from build123d import *

# Parameters (mm, degrees)
SKETCH1_W           = 38.1
SKETCH1_H           = 38.1
BOSS_EXTRUDE1_DEPTH = 61.087
SKETCH2_R           = 45.085
BOSS_EXTRUDE2_DEPTH = 3.175


with BuildPart() as part:
    # Sketch1 → Boss-Extrude1 (new body)
    with BuildSketch(Plane(origin=(0, 0, 0), x_dir=(1, 0, 0), z_dir=(0, 1, 0))):
        Rectangle(SKETCH1_W, SKETCH1_H)
    extrude(amount=BOSS_EXTRUDE1_DEPTH)

    # Sketch2 → Boss-Extrude2 (add)
    with BuildSketch(Plane.XZ):
        Circle(SKETCH2_R)
    extrude(amount=BOSS_EXTRUDE2_DEPTH)


solid = part.part
Here's how the part is built. I have some questions about the finished solid (model axes, mm). A direction names the side the tool comes from. Give positions to 0.01 mm unless a question says otherwise; leave off trailing zeros. Order: outer loops, then holes, each group sorted by start corner. A loop starts at its lowest first (then second) coordinate and runs counter-clockwise, first axis right, second up. Notation, with made-up numbers: M 69.25,4.25 L 75.25,4.25 A24 ccw 75.25,40.25 Z; hole C 66,29.25 d4. An arc over 180 degrees is marked long. Answer as a JSON object with one key per item and string values. Group by question number.
1) Suppose I cut it at B-B, the plane z = 0. Write out the boundary of the cut face in (x, y) (3 decimals), plus the area to 3 significant figures.
2) Suppose I cut it at A-A, the plane x = 0. Write out the boundary of the cut face in (y, z) (3 decimals), plus the area to 3 significant figures.
3) Please list where these lines run through material, in increasing order: L1, parallel to Y at x = 18, z = 30 (3 decimals); L2, parallel to Z at x = 7, y = 26. Write a range as [from, to].
4) On a 3-axis mill with a long thin cutter (end or side, diameter ignored), from which of +Z, -Z, +X, -X, +Y, -Y can I reach the whole of each face in a straight line? I mean faces 1 (the flat face through (19.05, 30, 0)), 2 (the flat face through (0, 30, 19.05)), 3 (the flat face through (-19.05, 30, 0)), 4 (the flat face through (0, 30, -19.05)). Say none if no direction works.
5) I'm going to push flat-ended pins straight in: pin 1 Ø2 at (y, z) = (34.5, 8.5) entering from +X; pin 2 Ø19 at (x, y) = (7, 31) entering from +Z; pin 3 Ø12 at (x, z) = (-25, 33) entering from +Y. Where does each tip first touch, or does it pass through?
6) Suppose I cut it at C-C, the plane y = 25. Write out the boundary of the cut face in (x, z), plus the area to 3 significant figures.
7) Suppose I cut it at D-D, the plane x = -22.5. Write out the boundary of the cut face in (y, z) (3 decimals), plus the area to 3 significant figures.
Results found:
{
 "1": {"outline": "M -45.085,-3.175 L 45.085,-3.175 L 45.085,0 L 19.05,0 L 19.05,61.087 L -19.05,61.087 L -19.05,0 L -45.085,0 Z", "area": "2,610 mm²"},
 "2": {"outline": "M -3.175,-45.085 L 0,-45.085 L 0,-19.05 L 61.087,-19.05 L 61.087,19.05 L 0,19.05 L 0,45.085 L -3.175,45.085 Z", "area": "2,610 mm²"},
 "3": {"L1": "[-3.175, 0]", "L2": "[-19.05, 19.05]"},
 "4": {"face 1": "+Z, -Z, +X, +Y", "face 2": "+Z, +X, -X, +Y", "face 3": "+Z, -Z, -X, +Y", "face 4": "-Z, +X, -X, +Y"},
 "5": {"pin 1": "x = 19.05", "pin 2": "z = 19.05", "pin 3": "y = 0"},
 "6": {"outline": "M -19.05,-19.05 L 19.05,-19.05 L 19.05,19.05 L -19.05,19.05 Z", "area": "1,450 mm²"},
 "7": {"outline": "M -3.175,-39.069 L 0,-39.069 L 0,39.069 L -3.175,39.069 Z", "area": "248 mm²"}
}
